```python
from build123d import *

# Parameters (mm, degrees)
CROQUIS1_R              = 5
SALIENTE_EXTRUIR1_DEPTH = 8
CROQUIS2_R              = 1.25
CORTAR_EXTRUIR1_DEPTH   = 6
CROQUIS3_R              = 2
SALIENTE_EXTRUIR2_DEPTH = 10
CHAFL_N1_SIZE           = 2


with BuildPart() as part:
    # Croquis1 → Saliente-Extruir1 (new body)
    with BuildSketch(Plane.XY):
        Circle(CROQUIS1_R)
    extrude(amount=SALIENTE_EXTRUIR1_DEPTH)

    # Croquis2 → Cortar-Extruir1 (cut)
    with BuildSketch(Plane(origin=(0, 0, 0), x_dir=(-1, 0, 0), z_dir=(0, 0, -1))):
        Circle(CROQUIS2_R)
    extrude(amount=-CORTAR_EXTRUIR1_DEPTH, mode=Mode.SUBTRACT)

    # Croquis3 → Saliente-Extruir2 (add)
    with BuildSketch(Plane.XY.offset(8)):
        Circle(CROQUIS3_R)
    extrude(amount=SALIENTE_EXTRUIR2_DEPTH)

    # Chaflán1
    chafl_n1_edges = [part.edges().sort_by_distance(p)[0] for p in [
        (-2, 0, 18),
    ]]
    chamfer(chafl_n1_edges, length=CHAFL_N1_SIZE)


solid = part.part
```
Input: part model. Units: mm. Frame: model coordinates. A direction names the side the tool comes from. Coordinates: 2 decimals unless noted, no trailing zeros. Order: outer loops, then holes, each group sorted by start corner. A loop starts at its lowest first (then second) coordinate and runs counter-clockwise, first axis right, second up. Notation, with made-up numbers: (65.5, -18.5) - (86.5, -18.5) arc R25 cw to (86.5, 1.5) - close; hole circle Ø6 at (51.25, 26). An arc over 180 degrees is marked (long way). Return JSON: item names as keys, results as strings.
Q1. Cut plane D-D (z = 9). Return loops of the section in (x, y).
The answers:
{"outline": "circle Ø4 at (0, 0)"}
Q2. Ray query, probe 1 along Y at (x, z) = (0, 4.2); probe 2 along Z at (x, y) = (-2.25, 1); probe 3 along Y at (x, z) = (-0.5, 4.5). Return the intervals inside material, ascending.
The answers:
{"probe 1": "y = -5 to -1.25, 1.25 to 5", "probe 2": "z = 0 to 8", "probe 3": "y = -4.97 to -1.15, 1.15 to 4.97"}
Q3. First-contact query: pin 1 (3 mm diameter, centred on x = -2, z = 9, fed in from +Y); pin 2 (5 mm diameter, centred on y = 3, z = 14.5, fed in from +X); pin 3 (6 mm diameter, centred on x = -3, z = 14, fed in from -Y). Flat tips, straight axial feed; report the tip coordinate or a pass-through.
The answers:
{"pin 1": "stops at y = 4.92", "pin 2": "stops at x = 1.94", "pin 3": "stops at y = -2"}
Q4. Access query for faces 1 (the cylindrical face through (0, -2, 12)), 2 (the flat face through (1, -1, 0)), 3 (the cylindrical face through (0.27, -1.22, 2.96)). Directions: +Z, -Z, +X, -X, +Y, -Y. A direction counts if a zero-diameter tool reaches every point of the face in a straight line with its end or side. Return the directions, or none.
The answers:
{"face 1": "+Z", "face 2": "-Z, +X, -X, +Y, -Y", "face 3": "-Z"}
Q5. Cut plane B-B (y = 3). Return loops of the section in (x, z), then the cut area to 3 significant figures.
The answers:
{"outline": "(-4, 0) - (4, 0) - (4, 8) - (-4, 8) - close", "area": "64.0 mm2"}
Q6. Cut plane A-A (z = 4.25). Return loops of the section in (x, y).
The answers:
{"outline": "circle Ø10 at (0, 0); hole circle Ø2.5 at (0, 0)"}
Q7. Draft query along X for faces 4 (the cylindrical face through (-1.08, -4.88, 3.94)), 5 (the flat face through (0, 0, 6)), 6 (the flat face through (-0.1, -2.2, 8)). Return one class per face: +X half, -X half, draft (parallel to the pull), parting line (faces both ways), or undercut.
The answers:
{"face 4": "parting line", "face 5": "undercut", "face 6": "draft"}
